Build history of the part. All positions in model axes, mm. A direction names the side the tool comes from. Give positions to 0.01 mm unless a question says otherwise; leave off trailing zeros. Write each loop counter-clockwise with the first axis right and the second up, starting at its lowest first coordinate (ties: lowest second). Pieces come first, ordered by that corner, then holes. Notation, with made-up numbers: (69.25, -2) -> (117.25, -2) arc R28 ccw to (117.25, 36) -> close; hole circle Ø5 at (6, -17.5). An arc over 180 degrees is marked (long way). Put each result on its own line as item: value. Start each with the question number.
Item 1: Slice it at C-C, the plane y = 1.75. List the corners of the cut face in (x, z).
Item 2: Tool access for faces 1 (the cylindrical face through (-0.1, 7.5, -7.5)), 2 (the cylindrical face through (5.087, 3.819, 4.327)), 3 (the cylindrical face through (-7.5, 7.5, 0.1)), 4 (the cylindrical face through (7.5, 7.5, -0.1)): list every direction of +Z, -Z, +X, -X, +Y, -Y with a clear straight run to the whole face (end or side of a thin tool).
Item 3: Slice it at D-D, the plane z = -8.5. List the corners of the cut face in (x, y), plus the area to 3 significant figures.
Item 4: Slice it at A-A, the plane y = 5.5. List the corners of the cut face in (x, z), plus the area to 3 significant figures.
Item 5: Drill centre lines: line 1 along Z through (x, y) = (4.5, 4.5); line 2 along Z through (x, y) = (6, 4.25); line 3 along Y through (x, z) = (-7.25, 4.75). Where is each one in solid material? Low to high.
Item 6: Flat gauge pins, fed straight in: pin 1 Ø4 at (y, z) = (6, 0.5) entering from +X; pin 2 Ø2 at (x, y) = (4, 5.5) entering from +Z; pin 3 Ø2 at (y, z) = (2.5, -4.5) entering from -X; pin 4 Ø1.8 at (x, z) = (5.3, 5.3) entering from -Y. Where does each tip first touch, or does it go through?
Item 7: Slice it at B-B, the plane x = 0. List the corners of the cut face in (y, z).
Item 8: Two-plate mould, pull along X, no slides. Class faces 5 (the cylindrical face through (4.566, 3.819, -4.627)), 6 (the flat face through (-4, 5, -7)), 7 (the cylindrical face through (0.1, 7.5, 7.5)): pulls with the +X half, pulls with the -X half, needs draft (parallel to the pull), parting line crosses it, or undercut.
Autodesk Inventor part; units mm, degrees
ref_plane "YZ Plane" through (0, 0, 0) normal (1, 0, 0) x (0, 1, 0)
ref_plane "XZ Plane" through (0, 0, 0) normal (0, 1, 0) x (-1, 0, 0)
ref_plane "XY Plane" through (0, 0, 0) normal (0, 0, 1) x (1, 0, 0)
sketch "Sketch1" plane through (0, 0, 0) normal (0, 1, 0) x (-1, 0, 0)
  circle A0 centre (0, 0) radius 10
  circle A1 centre (0, 0) radius 7.5
  dimension "d0" = 20
  dimension "d1" = 15
extrude "Extrusion1" add sketch "Sketch1" along normal blind 10 contours A1
extrude "Extrusion2" add sketch "Sketch1" along normal blind 5
sketch "Sketch2" plane through (0, 0, 0) normal (0, -1, 0) x (1, 0, 0)
  circle A0 centre (0, 0) radius 10
  line L0 (0, 0) -> (10, 0) construction
  line L1 (7.0711, -7.0711) -> (6.0104, -6.0104)
  circle A1 centre (0, 0) radius 7.5
  circle A2 centre (5.3033, 5.3033) radius 1
  line L2 (0, 0) -> (2.7588, 0)
  line L3 (0, 0) -> (0, -2.4662)
  circle A3 centre (5.3033, -5.3033) radius 1
  circle A4 centre (-5.3033, 5.3033) radius 1
  circle A5 centre (-5.3033, -5.3033) radius 1
  dimension "d7" = 2
extrude "Extrusion3" cut sketch "Sketch2" against normal blind 10 contours A3 A1 | A3 A1 | A5 A1 | A1 A5 | A2 A1 | A1 A2 | A4 A1 | A1 A4
properties part number "magnete"
Values follow:
1. outline: circle Ø20 at (0, 0); hole circle Ø2 at (-5.3, -5.3); hole circle Ø2 at (-5.3, 5.3); hole circle Ø2 at (5.3, -5.3); hole circle Ø2 at (5.3, 5.3)
2. face 1: -Z, +Y
2. face 2: +Y, -Y
2. face 3: -X, +Y
2. face 4: +X, +Y
3. outline: (-5.27, 0) -> (5.27, 0) -> (5.27, 5) -> (-5.27, 5) -> close
3. area: 52.7 mm2
4. outline: (-5.96, -4.55) arc R1 cw to (-4.55, -5.96) arc R7.5 ccw to (4.55, -5.96) arc R1 cw to (5.96, -4.55) arc R7.5 ccw to (5.96, 4.55) arc R1 cw to (4.55, 5.96) arc R7.5 ccw to (-4.55, 5.96) arc R1 cw to (-5.96, 4.55) arc R7.5 ccw to start
4. area: 171 mm2
5. line 1: -8.93 to -5.9, -4.71 to 4.71, 5.9 to 8.93
5. line 2: -8 to -6.02, -4.59 to 4.59, 6.02 to 8
5. line 3: 0 to 5
6. pin 1: x = 10
6. pin 2: z = 9.5
6. pin 3: x = -9.37
6. pin 4: through
7. outline: (0, -10) -> (5, -10) -> (5, -7.5) -> (10, -7.5) -> (10, 7.5) -> (5, 7.5) -> (5, 10) -> (0, 10) -> close
8. face 5: undercut
8. face 6: needs draft
8. face 7: parting line crosses it
